from build123d import *

# Parameters (mm, degrees)
PAD_DEPTH = 10


with BuildPart() as part:
    # Sketch → Pad (new body)
    with BuildSketch(Plane.XY):
        with BuildLine():
            ThreePointArc((8.291561, 12.500001), (10.081337, 5.820463), (14.971099, 0.930702))
            ThreePointArc((6.679538, -13.430703), (20.49038, -11.830126), (14.971099, 0.930702))
            ThreePointArc((6.679538, -13.430703), (0, -11.640926), (-6.679538, -13.430703))
            ThreePointArc((-14.971099, 0.930702), (-20.49038, -11.830126), (-6.679538, -13.430703))
            ThreePointArc((-14.971099, 0.930702), (-10.081337, 5.820463), (-8.291561, 12.500001))
            ThreePointArc((8.291561, 12.500001), (0, 23.660253), (-8.291561, 12.500001))
        make_face()
        with BuildLine():
            ThreePointArc((-6.5, 0), (-5.230811, 1.699593), (-5.25861, 3.820604))
            ThreePointArc((-5.25861, 3.820604), (-3.232819, 4.449593), (-2.00861, 6.181867))
            ThreePointArc((-2.00861, 6.181867), (0, 5.5), (2.00861, 6.181867))
            ThreePointArc((2.00861, 6.181867), (3.232819, 4.449593), (5.25861, 3.820604))
            ThreePointArc((5.25861, 3.820604), (5.230811, 1.699593), (6.5, 0))
            ThreePointArc((6.5, 0), (5.230811, -1.699593), (5.25861, -3.820604))
            ThreePointArc((5.25861, -3.820604), (3.232819, -4.449593), (2.00861, -6.181867))
            ThreePointArc((2.00861, -6.181867), (0, -5.5), (-2.00861, -6.181867))
            ThreePointArc((-2.00861, -6.181867), (-3.232819, -4.449593), (-5.25861, -3.820604))
            ThreePointArc((-5.25861, -3.820604), (-5.230811, -1.699593), (-6.5, 0))
        make_face(mode=Mode.SUBTRACT)
    extrude(amount=PAD_DEPTH)


solid = part.part
Verification items for the finished model (mm, model axes). A direction names the side the tool comes from. Give positions to 0.01 mm unless a question says otherwise; leave off trailing zeros. Loops run counter-clockwise (first coordinate to the right, second up) from the corner with the lowest first, then second, coordinate; pieces in that order, holes last.
1. Cross-section at A-A on z = 4.75. Record the cut outline in (x, y), and give its area (3 significant figures).
Derived:
outline: (-14.97, 0.93) arc R8.66 ccw (long way) to (-6.68, -13.43) arc R13.36 cw to (6.68, -13.43) arc R8.66 ccw (long way) to (14.97, 0.93) arc R13.36 cw to (8.29, 12.5) arc R8.66 ccw (long way) to (-8.29, 12.5) arc R13.36 cw to start; hole (-6.5, 0) arc R3.3 cw to (-5.26, -3.82) arc R3.3 cw to (-2.01, -6.18) arc R3.3 cw to (2.01, -6.18) arc R3.3 cw to (5.26, -3.82) arc R3.3 cw to (6.5, 0) arc R3.3 cw to (5.26, 3.82) arc R3.3 cw to (2.01, 6.18) arc R3.3 cw to (-2.01, 6.18) arc R3.3 cw to (-5.26, 3.82) arc R3.3 cw to start
area: 908 mm2
2. Cross-section at C-C on y = 15. Record the cut outline in (x, z).
Derived:
outline: (-8.66, 0) - (8.66, 0) - (8.66, 10) - (-8.66, 10) - close
3. Cross-section at B-B on x = 0. Record the cut outline in (y, z).
Derived:
outline: (-11.64, 0) - (-5.5, 0) - (-5.5, 10) - (-11.64, 10) - close; (5.5, 0) - (23.66, 0) - (23.66, 10) - (5.5, 10) - close
4. Release check for a two-part mould opening along Y. For faces 1 (the flat face through (-5, 4, 0)), 2 (the cylindrical face through (20.375, -12.024, 4.93)), 3 (the cylindrical face through (-3.208, -4.467, 4.93)) record: +Y half, -Y half, draft (parallel to the pull), parting line (faces both ways), or undercut.
Derived:
face 1: draft
face 2: parting line
face 3: undercut
5. Material ranges on probe 1 along X at (y, z) = (6, 8.25); probe 2 along Y at (x, z) = (0, 6.5); probe 3 along X at (y, z) = (-1.5, 2), recorded low to high.
Derived:
probe 1: x = -9.98 to -2.07, -1.75 to 1.75, 2.07 to 9.98
probe 2: y = -11.64 to -5.5, 5.5 to 23.66
probe 3: x = -19.24 to -5.3, 5.3 to 19.24
6. Go/stop test with flat-tipped pins: P1, Ø2, axis at y = 19.5, z = 7, coming from the +X side; P2, Ø5, axis at x = -7, z = 3.5, coming from the +Y side; P3, Ø4, axis at x = -17, z = 5, coming from the -Y side. Record where each tip stops, or that it passes through.
Derived:
P1: stops at x = 7.92
P2: stops at y = 22.4
P3: stops at y = -15.92
7. Tool access check on faces 4 (the cylindrical face through (10.03, 5.91, 4.93)), 5 (the cylindrical face through (-10.13, 5.74, 4.93)), 6 (the cylindrical face through (0.226, 23.657, 4.93)). Record the directions out of +Z, -Z, +X, -X, +Y, -Y that give a thin tool (end or side, any length) a straight path to the whole face; none if there is none.
Derived:
face 4: +Z, -Z, +X
face 5: +Z, -Z, -X
face 6: +Z, -Z
8. Cross-section at D-D on x = -18. Record the cut outline in (y, z).
Derived:
outline: (-14.56, 0) - (-0.44, 0) - (-0.44, 10) - (-14.56, 10) - close
